Could you check a few things on this model? Use its own coordinates, in mm. A direction names the side the tool comes from. Round coordinates to 2 decimals unless told otherwise and drop trailing zeros. Order: outer loops, then holes, each group sorted by start corner. A loop starts at its lowest first (then second) coordinate and runs counter-clockwise, first axis right, second up. Notation, with made-up numbers: (-30, 56.5) - (-4, 56.5) arc R26 cw to (-4, 85.5) - close; hole circle Ø10 at (70.25, 14). An arc over 180 degrees is marked (long way). Use one line per item in the form item = value.
from build123d import *

# Parameters (mm, degrees)
SKETCH2_R           = 20
BOSS_EXTRUDE1_DEPTH = 30
SKETCH6_R           = 7.5
BOSS_EXTRUDE3_DEPTH = 40
SKETCH7_R           = 3
CUT_EXTRUDE1_DEPTH  = 49.989794856
CHAMFER1_SIZE       = 1.5


# Read off the part's stored shape, not the designer's step: M3 Tapped Hole1
with BuildPart() as part:
    # Sketch2 → Boss-Extrude1 (new body)
    with BuildSketch(Plane(origin=(0, 0, 0), x_dir=(1, 0, 0), z_dir=(0, 1, 0))):
        with Locations(Location((0, 0, 0), (0, 0, 270))):
            Circle(SKETCH2_R)
    extrude(amount=BOSS_EXTRUDE1_DEPTH)

    # Sketch6 → Boss-Extrude3 (add)
    with BuildSketch(Plane(origin=(0, 0, 0), x_dir=(1, 0, 0), z_dir=(0, 1, 0))):
        with Locations(Location((0, 0, 0), (0, 0, 270))):
            Circle(SKETCH6_R)
    extrude(amount=BOSS_EXTRUDE3_DEPTH)

    # Sketch7 → Cut-Extrude1 (cut, through all)
    with BuildSketch(Plane(origin=(0, 40, 0), x_dir=(1, 0, 0), z_dir=(0, 1, 0))):
        with Locations(Location((0, 0, 0), (0, 0, 270))):
            Circle(SKETCH7_R)
    extrude(amount=-CUT_EXTRUDE1_DEPTH, mode=Mode.SUBTRACT)

    # M3 Tapped Hole1 outline → M3 Tapped Hole1 (revolve, cut)
    with BuildSketch(Plane(origin=(0, 35, 0), x_dir=(0, 1, 0), z_dir=(0, 0, -1))):
        Polygon((1.525048793, 7.500048793), (0, 7.500048793), (0, 2.72705461), (1.25, 2.72705461), (1.25, 7.225), align=None)
    revolve(axis=Axis((0, 35, 0), (1, 0, 0)), mode=Mode.SUBTRACT)

    # Chamfer1
    chamfer1_edges = [part.edges().sort_by_distance(p)[0] for p in [
        (0, 0, -20),
        (0, 30, -20),
    ]]
    chamfer(chamfer1_edges, length=CHAMFER1_SIZE)


solid = part.part
Item 1: For faces 4 (the face through (0, 0, 4)), 5 (the face through (-7.32, 34.93, -1.63)), 6 (the face through (5.01, 34.01, -0.76)), which set-ups out of +Z, -Z, +X, -X, +Y, -Y let a thin tool reach every point of the face, with its end or its side?
Found:
face_4 = +Z, -Z, +X, -X, -Y
face_5 = +Y
face_6 = +X
Item 2: Will these pins go through, and if not, where does the flat tip stop? P1, Ø2, axis at y = 25.5, z = 2, coming from the +X side (3 decimals); P2, Ø8, axis at y = 11.5, z = -4, coming from the -X side; P3, Ø12, axis at y = 22, z = -11, coming from the +X side.
Found:
P1 = 19.975
P2 = -20
P3 = 19.36
Item 3: Imagine slicing it at D-D on y = 35. Please give me the cut outline in (x, z) (3 decimals).
Found:
outline = (2.727, -1.25) arc R3 cw (long way) to (2.727, 1.25) - (7.225, 1.25) - (7.369, 1.394) arc R7.5 ccw (long way) to (7.369, -1.394) - (7.225, -1.25) - close
Item 4: Imagine slicing it at C-C on y = 5. Please give me the cut outline in (x, z).
Found:
outline = circle Ø40 at (0, 0); hole circle Ø6 at (0, 0)
Item 5: If we mould it in two halves opening along Z, with no side actions, what happens to faces 1 (the face through (-19.524, 14.811, -4.336)), 2 (the face through (0.9, 20.28, 2.86)), 3 (the face through (0, 30, 8))? For each: released by +Z, released by -Z, zero draft, split by the parting line, or undercut.
Found:
face_1 = split by the parting line
face_2 = undercut
face_3 = zero draft
Item 6: Imagine slicing it at B-B on z = 0. Please give me the cut outline in (x, y) (3 decimals).
Found:
outline = (-20, 1.5) - (-18.5, 0) - (-3, 0) - (-3, 40) - (-7.5, 40) - (-7.5, 30) - (-18.5, 30) - (-20, 28.5) - close; (3, 0) - (18.5, 0) - (20, 1.5) - (20, 28.5) - (18.5, 30) - (7.5, 30) - (7.5, 33.475) - (7.225, 33.75) - (3, 33.75) - close; (3, 36.25) - (7.225, 36.25) - (7.5, 36.525) - (7.5, 40) - (3, 40) - close
Item 7: I need wall thicknesses on L1, parallel to X at y = 20, z = 0; L2, parallel to Y at x = 5, z = 0; L3, parallel to Y at x = -15, z = 2. Which ranges of each line are inside material? Lowest first, please.
Found:
L1 = -20 to -3, 3 to 20
L2 = 0 to 33.75, 36.25 to 40
L3 = 0 to 30
Item 8: Imagine slicing it at A-A on x = 0. Please give me the cut outline in (y, z), plus the area to 3 significant figures.
Found:
outline = (0, -18.5) - (1.5, -20) - (28.5, -20) - (30, -18.5) - (30, -7.5) - (40, -7.5) - (40, -3) - (0, -3) - close; (0, 3) - (40, 3) - (40, 7.5) - (30, 7.5) - (30, 18.5) - (28.5, 20) - (1.5, 20) - (0, 18.5) - close
area = 1,110 mm2
